from build123d import *

# Parameters (mm, degrees)
F1_DEPTH = 19.05


with BuildPart() as f1:
    # F0 (on Front) → F1 (new body)
    with BuildSketch(Plane.XZ):
        with BuildLine():
            Line((101.6, 76.2), (-127, 76.2))
            Line((-127, 76.2), (-127, -76.2))
            Line((-127, -76.2), (-114.3, -76.2))
            ThreePointArc((-114.3, -76.2), (-107.345229, -42.151908), (-88.9, -12.7))
            Line((-88.9, -12.7), (101.6, 25.4))
            ThreePointArc((101.6, 25.4), (118.145251, 34.254749), (127, 50.8))
            ThreePointArc((127, 50.8), (119.560512, 68.760512), (101.6, 76.2))
        make_face()
    extrude(amount=F1_DEPTH)


solid = f1.part
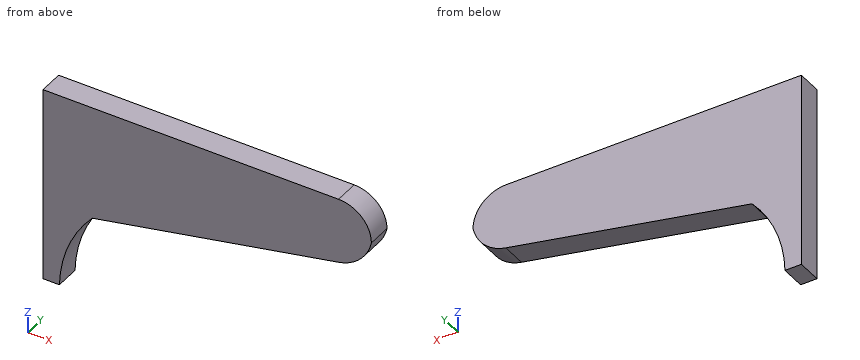
Could you check a few things on this model? Use its own coordinates, in mm. Round coordinates to 2 decimals unless told otherwise and drop trailing zeros. Order: outer loops, then holes, each group sorted by start corner. A loop starts at its lowest first (then second) coordinate and runs counter-clockwise, first axis right, second up.
(1) Please list where these lines run through material, in increasing order: line 1 along Z through (x, y) = (68.5, -15.5); line 2 along Z through (x, y) = (115.5, -14.5); line 3 along X through (y, z) = (-16.5, -30).
Response values:
line 1: z = 18.78 to 76.2
line 2: z = 31.88 to 72.06
line 3: x = -127 to -101.48
(2) I'm going to push flat-ended pins straight in: pin 1 (2 mm diameter, centred on x = 98, y = -4.5, fed in from -Z); pin 2 (2 mm diameter, centred on x = -94, y = -9, fed in from -Z); pin 3 (3 mm diameter, centred on y = -4, z = -34, fed in from +X). Where does each tip first touch, or does it pass through?
Response values:
pin 1: stops at z = 24.48
pin 2: stops at z = -20.1
pin 3: stops at x = -102.86
(3) Imagine slicing it at C-C (x = 97). Write out the boundary of the cut face in (y, z), plus the area to 3 significant figures.
Response values:
outline: (-19.05, 24.48) - (0, 24.48) - (0, 76.2) - (-19.05, 76.2) - close
area: 985 mm2
(4) Imagine slicing it at B-B (z = 10). Write out the boundary of the cut face in (x, y).
Response values:
outline: (-127, -19.05) - (24.6, -19.05) - (24.6, 0) - (-127, 0) - close
(5) Imagine slicing it at A-A (y = -16.25). Write out the boundary of the cut face in (x, z), plus the area to 3 significant figures.
Response values:
outline: (-127, -76.2) - (-114.3, -76.2) arc R97.58 cw to (-88.9, -12.7) - (101.6, 25.4) arc R32.38 ccw to (127, 50.8) arc R25.4 ccw to (101.6, 76.2) - (-127, 76.2) - close
area: 19,000 mm2
